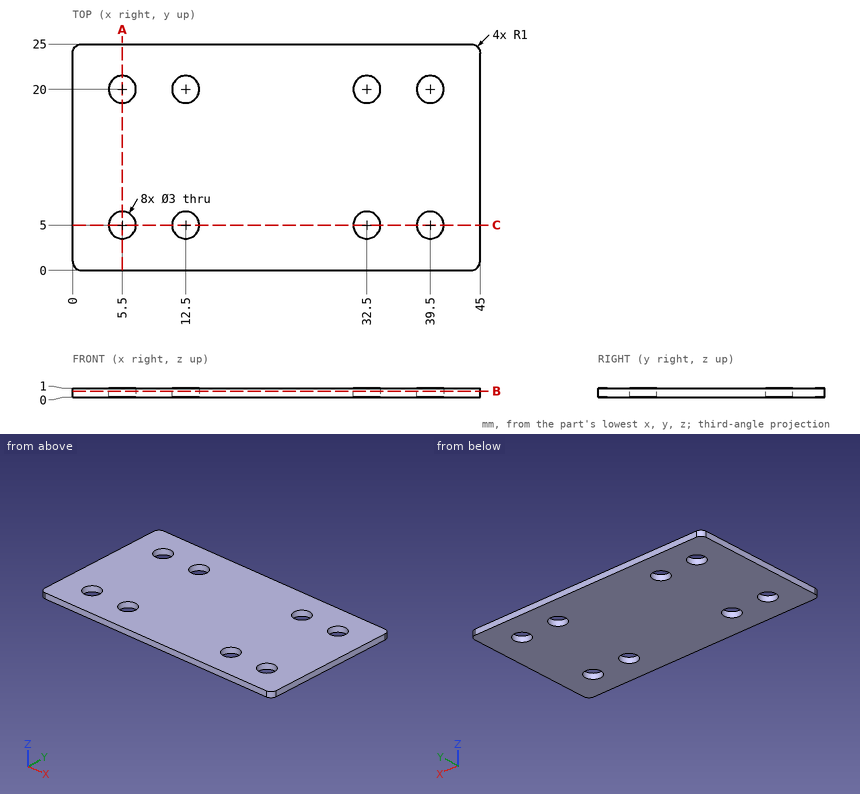
Can you work these out from the drawing? Everything is in mm from the part's minimum corner. Coordinates: 2 decimals unless noted, no trailing zeros. Order: outer loops, then holes, each group sorted by start corner. A loop starts at its lowest first (then second) coordinate and runs counter-clockwise, first axis right, second up. Notation, with made-up numbers: (18, 16) -> (42, 16) arc R24 ccw to (42, 49) -> close; hole circle Ø9 at (-26.75, 82.5). An arc over 180 degrees is marked (long way). Return JSON: item names as keys, results as strings.
1) If I drill on probe 1 along Y at (x, z) = (39.5, 0.4), over which ranges is the centre line in solid material (lowest first)?
Conclusion:
{"probe 1": "y = 0 to 3.5, 6.5 to 18.5, 21.5 to 25"}
2) If we section it at C-C on y = 5: List the corners of the cut face in (x, z) for me.
Conclusion:
{"outline": "(0, 0) -> (4, 0) -> (4, 1) -> (0, 1) -> close; (7, 0) -> (11, 0) -> (11, 1) -> (7, 1) -> close; (14, 0) -> (31, 0) -> (31, 1) -> (14, 1) -> close; (34, 0) -> (38, 0) -> (38, 1) -> (34, 1) -> close; (41, 0) -> (45, 0) -> (45, 1) -> (41, 1) -> close"}
3) If we section it at A-A on x = 5.5: List the corners of the cut face in (y, z) for me.
Conclusion:
{"outline": "(0, 0) -> (3.5, 0) -> (3.5, 1) -> (0, 1) -> close; (6.5, 0) -> (18.5, 0) -> (18.5, 1) -> (6.5, 1) -> close; (21.5, 0) -> (25, 0) -> (25, 1) -> (21.5, 1) -> close"}
4) I'm going to push a flat-ended pin straight in: P1, Ø3.5, axis at x = 32.5, y = 5, coming from the +Z side. Where does the tip first touch, or does it pass through?
Conclusion:
{"P1": "stops at z = 1"}
5) If we section it at B-B on z = 0.7: State how many separate pieces and enclosed holes the cut face has, plus the area to 3 significant figures.
Conclusion:
{"separate pieces": "1", "enclosed holes": "8", "area": "1,070 mm²"}
